Autodesk Inventor part; units mm, degrees
ref_plane "YZ Plane" through (0, 0, 0) normal (1, 0, 0) x (0, 1, 0)
ref_plane "XZ Plane" through (0, 0, 0) normal (0, 1, 0) x (-1, 0, 0)
ref_plane "XY Plane" through (0, 0, 0) normal (0, 0, 1) x (1, 0, 0)
sketch "Sketch1" plane through (0, 0, 0) normal (0, 0, 1) x (1, 0, 0)
  line L0 (-36.6197, 6.2354) -> (-25.8247, 6.2354)
  line L1 (-25.8247, 6.2354) -> (-25.8247, -22.3396)
  line L2 (-25.8247, -22.3396) -> (-36.6197, -22.3396)
  line L3 (-36.6197, -22.3396) -> (-36.6197, 6.2354)
  line L4 (-25.8247, 3.0604) -> (-19.4747, 3.0604)
  line L5 (-19.4747, 3.0604) -> (-14.9147, -3.2896)
  line L6 (-14.9147, -3.2896) -> (26.9953, -3.2896)
  line L7 (26.9953, -3.2896) -> (26.9953, -22.3396)
  line L8 (26.9953, -22.3396) -> (-25.8247, -22.3396)
  point P0 (0, 0)
  dimension "d0" = 28.575
  dimension "d1" = 10.795
  dimension "d2" = 25.4
  dimension "d3" = 19.05
  dimension "d4" = 41.91
  dimension "d5" = 6.35
extrude "Extrusion1" add sketch "Sketch1" along normal blind 10.16
sketch "Sketch2" plane through (0, 0, 0) normal (0, 0, -1) x (-1, 0, 0)
  line L0 (36.6197, -22.3396) -> (-26.9953, -22.3396)
  line L1 (36.6197, 6.2354) -> (25.8247, 6.2354)
  line L2 (25.8247, 6.2354) -> (25.8247, -22.3396)
  line L3 (25.8247, -22.3396) -> (36.6197, -22.3396)
  line L4 (36.6197, -22.3396) -> (36.6197, 6.2354)
  point P0 (0, 0)
extrude "Extrusion2" add sketch "Sketch2" along normal blind 0.254
sketch "Sketch3" plane through (0, 0, 10.16) normal (0, 0, 1) x (1, 0, 0)
  line L0 (26.9953, -22.3396) -> (-36.6197, -22.3396)
  line L1 (-36.6197, 6.2354) -> (-25.8247, 6.2354)
  line L2 (-25.8247, 6.2354) -> (-25.8247, -22.3396)
  line L3 (-25.8247, -22.3396) -> (-36.6197, -22.3396)
  line L4 (-36.6197, -22.3396) -> (-36.6197, 6.2354)
  point P0 (0, 0)
extrude "Extrusion3" add sketch "Sketch3" along normal blind 0.254
sketch "Sketch4" plane through (-25.8247, -22.3396, 0) normal (0, -1, 0) x (1, 0, 0)
  line L0 (-10.795, 10.414) -> (0, 10.414)
  line L1 (0, 10.414) -> (0, -0.254)
  line L2 (0, -0.254) -> (-10.795, -0.254)
  line L3 (-10.795, -0.254) -> (-10.795, 10.414)
  point P0 (25.8247, 0)
extrude "Extrusion4" add sketch "Sketch4" along normal blind 0.254
properties part number "Selenoid Part 1764"
Build history of the part. All positions in model axes, mm. A direction names the side the tool comes from. Round coordinates to 2 decimals unless told otherwise and drop trailing zeros. Write each loop counter-clockwise with the first axis right and the second up, starting at its lowest first coordinate (ties: lowest second). Pieces come first, ordered by that corner, then holes. Notation, with made-up numbers: (68, -30) - (87, -30) arc R18 cw to (87, -4) - close; hole circle Ø8 at (43.25, 88.25). An arc over 180 degrees is marked (long way). Write each question's results on one line, items separated by ' | '. Start each with the question number.
Item 1: Which spindle directions (+Z, -Z, +X, -X, +Y, -Y) get a long thin tool onto all of the face, cutting with end or side? Do faces 1 (the face through (1, -22.34, 5)), 2 (the face through (-36.62, -8, 5)), 3 (the face through (0, -12, 10.16)), 4 (the face through (0, -12, 0)), 5 (the face through (-23, 3.06, 5)). Say none if no direction does.
Item 2: Saw through at D-D (x = -23). Write the cut outline in (y, z), and give its area (3 significant figures).
Item 3: Drop flat-ended pins along their axis: P1, Ø3, axis at x = -3.5, z = 4.5, coming from the +Y side; P2, Ø7.5, axis at x = -0.5, y = -12, coming from the +Z side; P3, Ø1.9, axis at x = -21.5, z = 4.5, coming from the +Y side. Give the stop position or say it passes through.
Item 4: Saw through at B-B (z = 4.25). Write the cut outline in (x, y).
Item 5: Wall check: L1, parallel to Z at x = 8, y = -11.25; L2, parallel to Y at x = -4.5, z = 3.25; L3, parallel to X at y = 4, z = 3.5. Give the ranges that are in metal, low to high. Write a range as [from, to].
Item 6: Saw through at C-C (x = 8.5). Write the cut outline in (y, z), and give its area (3 significant figures).
Item 7: Saw through at A-A (y = -15). Write the cut outline in (x, z).
Results are:
1) face 1: +Z, -Z, +X, -Y | face 2: +Z, -Z, -X, +Y, -Y | face 3: +Z, +X, +Y, -Y | face 4: -Z, +X, +Y, -Y | face 5: +Z, -Z, +X, +Y
2) outline: (-22.34, 0) - (3.06, 0) - (3.06, 10.16) - (-22.34, 10.16) - close | area: 258 mm²
3) P1: stops at y = -3.29 | P2: stops at z = 10.16 | P3: stops at y = 3.06
4) outline: (-36.62, -22.59) - (-25.82, -22.59) - (-25.82, -22.34) - (27, -22.34) - (27, -3.29) - (-14.91, -3.29) - (-19.47, 3.06) - (-25.82, 3.06) - (-25.82, 6.24) - (-36.62, 6.24) - close
5) L1: z = [0, 10.16] | L2: y = [-22.34, -3.29] | L3: x = [-36.62, -25.82]
6) outline: (-22.34, 0) - (-3.29, 0) - (-3.29, 10.16) - (-22.34, 10.16) - close | area: 194 mm²
7) outline: (-36.62, -0.25) - (-25.82, -0.25) - (-25.82, 0) - (27, 0) - (27, 10.16) - (-25.82, 10.16) - (-25.82, 10.41) - (-36.62, 10.41) - close
